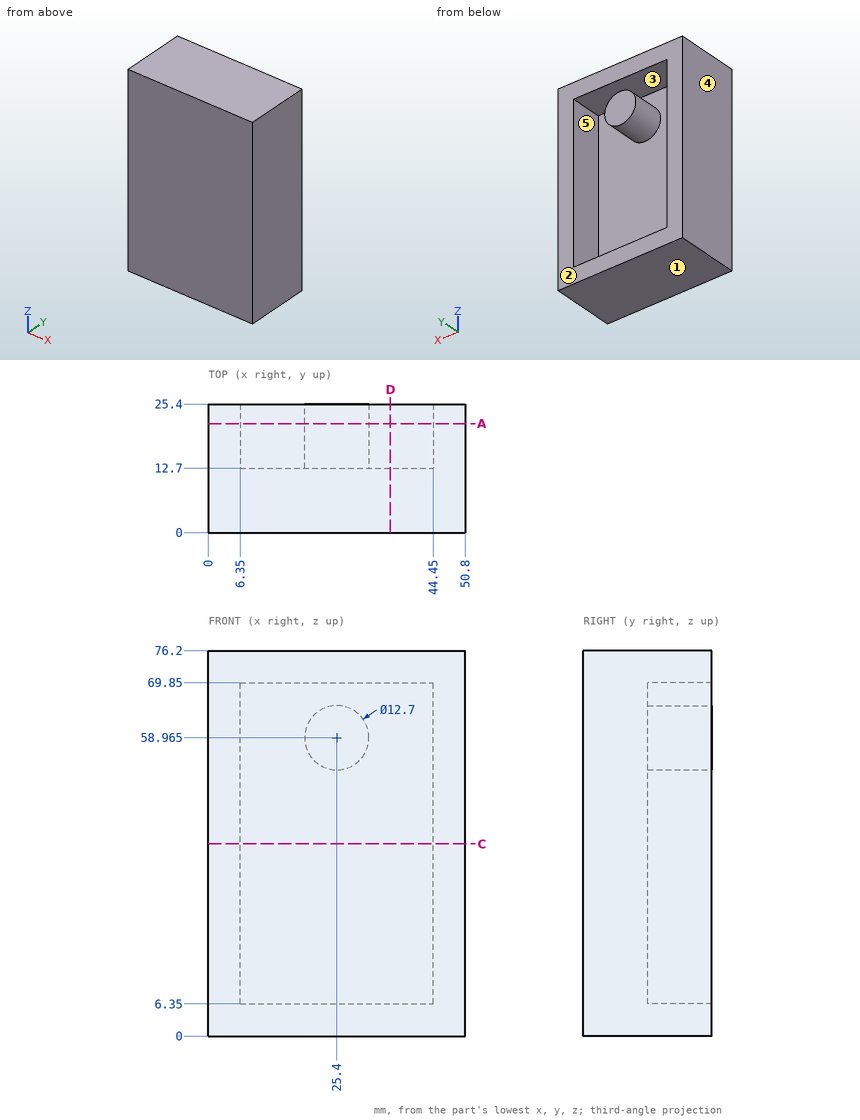
Drawing for the job (mm, zero at the part's lowest x, y, z). A direction names the side the tool comes from. Coordinates: 2 decimals unless noted, no trailing zeros. Order: outer loops, then holes, each group sorted by start corner. A loop starts at its lowest first (then second) coordinate and runs counter-clockwise, first axis right, second up. Notation, with made-up numbers: (-9.75, -20) - (-3.75, -20) arc R25 cw to (-3.75, 15) - close; hole circle Ø3 at (30, -36.75). An arc over 180 degrees is marked (long way). Use a Markdown table: item, result. Add a question column.
(1) Flat gauge pin, fed straight in: pin 1 (1.5 mm diameter, centred on x = 14, z = 28.5, fed in from +Y). Where does the tip first touch, or does it go through?
(2) Saw through at D-D (x = 36). Give the cut face in (y, z), then the cut area to 3 significant figures.
(3) Saw through at A-A (y = 21.5). Count the separate pieces of the cut face and the enclosed holes in it, then the cut area to 3 significant figures.
(4) Drill centre lines: line 1 along Z through (x, y) = (15.5, 23.5); line 2 along X through (y, z) = (23.5, 69.5); line 3 along Y through (x, z) = (32, 23). Where is each one in solid material? Low to high. Write a range as [from, to].
(5) Saw through at C-C (z = 38). Give the cut face in (x, y).
(6) Pull direction Z, two halves, no side cores. Call the marked faces 1, 2 and 3: +Z half, -Z half, draft (parallel to the pull), parting line (faces both ways), or undercut.
(7) Which spindle directions (+Z, -Z, +X, -X, +Y, -Y) get a long thin tool onto all of the face, cutting with end or side? Do the marked faces 4 and 5. Say none if no direction does.
Solved:
| question | item | result |
|---|---|---|
| 1 | pin 1 | stops at y = 12.7 |
| 2 | outline | (0, 0) - (25.4, 0) - (25.4, 6.35) - (12.7, 6.35) - (12.7, 69.85) - (25.4, 69.85) - (25.4, 76.2) - (0, 76.2) - close |
| 2 | area | 1,130 mm² |
| 3 | separate pieces | 2 |
| 3 | enclosed holes | 1 |
| 3 | area | 1,580 mm² |
| 4 | line 1 | z = [0, 6.35], [69.85, 76.2] |
| 4 | line 2 | x = [0, 6.35], [44.45, 50.8] |
| 4 | line 3 | y = [0, 12.7] |
| 5 | outline | (0, 0) - (50.8, 0) - (50.8, 25.4) - (44.45, 25.4) - (44.45, 12.7) - (6.35, 12.7) - (6.35, 25.4) - (0, 25.4) - close |
| 6 | face 1 | -Z half |
| 6 | face 2 | draft |
| 6 | face 3 | undercut |
| 7 | face 4 | +Z, -Z, -X, +Y, -Y |
| 7 | face 5 | +Y |
